```python
from build123d import *

# Parameters (mm, degrees)
F0_W     = 3
F0_H     = 30
F1_DEPTH = 3
F2_W     = 69
F2_H     = 57.5
F3_DEPTH = 25


with BuildPart() as f1:
    # F0 (on Right) → F1 (new body)
    with BuildSketch(Plane.YZ):
        Polygon((-89, 0), (0, 0), (0, 88.5), (0, 118.5), (0, 143.5), (-89, 143.5), (-89, 118.5), (-89, 88.5), align=None)
        with Locations((1.5, 103.5)):
            Rectangle(F0_W, F0_H)
        with Locations((-90.5, 103.5)):
            Rectangle(F0_W, F0_H)
    extrude(amount=F1_DEPTH)

    # F2 (on face) → F3 (cut)
    with BuildSketch(Plane.YZ.offset(3)):
        with Locations((-44.5, 95.75)):
            Rectangle(F2_W, F2_H)
    extrude(amount=-F3_DEPTH, mode=Mode.SUBTRACT)


solid = f1.part
```
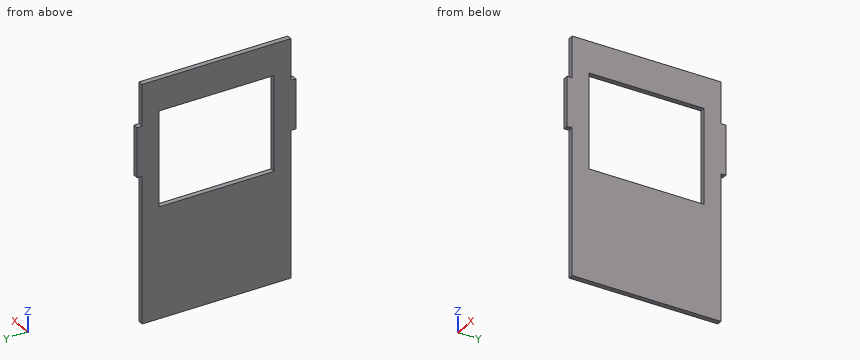
Source: CAD feature listing. Evaluate the final solid. Frame: model axes, mm. Round coordinates to 2 decimals unless told otherwise and drop trailing zeros. Write each loop counter-clockwise with the first axis right and the second up, starting at its lowest first coordinate (ties: lowest second). Pieces come first, ordered by that corner, then holes. Notation, with made-up numbers: M 3,-36.75 L 17,-36.75 A25 ccw 17,2.25 Z; hole C 75.5,-25.5 d8. An arc over 180 degrees is marked long. Use CSV: the item, a comma, the result in double quotes. Start each with the question number.
Q1. Cut plane D-D on z = 17. Output: boundary loops of the cut face in (x, y), plus the area to 3 significant figures.
Q2. Line query: line 1 (Z direction, x = 0.1, y = -49.5); line 2 (Y direction, x = 0.6, z = 104.5); line 3 (Y direction, x = 0.7, z = 30.5). Output: solid intervals per line, ascending. Write a range as from..to.
Q3. Cut plane C-C on x = 1.4. Output: boundary loops of the cut face in (y, z), plus the area to 3 significant figures.
Q4. Cut plane B-B on y = -17. Output: boundary loops of the cut face in (x, z).
Q5. Cut plane A-A on z = 84. Output: boundary loops of the cut face in (x, y).
Q6. First-contact query: P1, Ø1.5, axis at x = 1, z = 134.5, coming from the -Y side; P2, Ø1.5, axis at x = 1, y = -90.5, coming from the +Z side; P3, Ø1.5, axis at x = 2, y = -90, coming from the -Z side. Flat tips, straight axial feed; report the tip coordinate or a pass-through.
Results found:
1,outline,"M 0,-89 L 3,-89 L 3,0 L 0,0 Z"
1,area,"267 mm^2"
2,line 1,"0..67, 124.5..143.5"
2,line 2,"-92..-79, -10..3"
2,line 3,"-89..0"
3,outline,"M -92,88.5 L -89,88.5 L -89,0 L 0,0 L 0,88.5 L 3,88.5 L 3,118.5 L 0,118.5 L 0,143.5 L -89,143.5 L -89,118.5 L -92,118.5 Z; hole M -79,67 L -10,67 L -10,124.5 L -79,124.5 Z"
3,area,"8,980 mm^2"
4,outline,"M 0,0 L 3,0 L 3,67 L 0,67 Z; M 0,124.5 L 3,124.5 L 3,143.5 L 0,143.5 Z"
5,outline,"M 0,-89 L 3,-89 L 3,-79 L 0,-79 Z; M 0,-10 L 3,-10 L 3,0 L 0,0 Z"
6,P1,"y = -89"
6,P2,"z = 118.5"
6,P3,"z = 88.5"
